Autodesk Inventor part; units mm, degrees
ref_plane "Plan de construction1" through (0, 5, 0) normal (0, -1, 0) x (1, 0, 0)
ref_plane "YZ Plane" through (0, 0, 0) normal (1, 0, 0) x (0, 1, 0)
ref_plane "XZ Plane" through (0, 0, 0) normal (0, 1, 0) x (-1, 0, 0)
sketch "Esquisse1" plane through (0, 0, 0) normal (0, 1, 0) x (-1, 0, 0)
  circle A0 centre (0, 0) radius 17.75
  dimension "d0" = 35.5
extrude "Extrusion1" add sketch "Esquisse1" along normal blind 8
ref_plane "Plan de construction1" through (0, 5, 0) normal (0, -1, 0) x (1, 0, 0)
sketch "Esquisse2" plane through (0, 5, 0) normal (0, -1, 0) x (1, 0, 0)
  circle A0 centre (0, 0) radius 17.75 construction
  line L0 (0, 0) -> (11, 0) construction
  circle A1 centre (11, 0) radius 1.65
  dimension "d4" = 11
  dimension "d5" = 3.3
extrude "Extrusion2" cut sketch "Esquisse2" along normal through all both and the other way through all
sketch "Esquisse3" plane through (0, 5, 0) normal (0, -1, 0) x (1, 0, 0)
  line L0 (23.2, 2.825) -> (8.2, 2.825)
  line L1 (8.2, 2.825) -> (8.2, -2.825)
  line L2 (8.2, -2.825) -> (23.2, -2.825)
  line L3 (23.2, -2.825) -> (23.2, 2.825)
  circle A0 centre (11, 0) radius 1.65 construction
  circle A1 centre (0, 0) radius 17.75 construction
  line L4 (0, 0) -> (8.2, 0) construction
  dimension "d8" = 5.65
  dimension "d9" = 2.8
  dimension "d10" = 15
pattern_circular "Réseau circulaire1" count 3 over 360 about axis through (0, 0, 0) along (0, -1, 0) of "Extrusion2"
ref_plane "Work Plane2" through (0, 6.5, 0) normal (0, 1, 0) x (1, 0, 0)
sketch "Sketch4" plane through (0, 6.5, 0) normal (0, 1, 0) x (1, 0, 0)
  circle A0 centre (0, 0) radius 17
  circle A1 centre (-5.5, -9.5263) radius 1.65
  circle A2 centre (11, 0) radius 1.65
  circle A3 centre (0, 0) radius 17.75
  circle A4 centre (0, 0) radius 17.75
  line L0 (-5.1051, -17) -> (-5.1051, 17)
  dimension "d17" = 34
extrude "Extrusion4" [suppressed]
sketch "Sketch7" plane through (0, 0, 0) normal (0, -1, 0) x (1, 0, 0)
  circle A0 centre (-5.5, -9.5263) radius 1.65
  circle A1 centre (-5.5, 9.5263) radius 1.65
  circle A2 centre (11, 0) radius 1.65
  circle A3 centre (0, 0) radius 17.75
  arc A4 (12.2653, -21.0869) -> (-1.702, -23.304) centre (6.3902, -29.1791) ccw construction
  line L0 (12.2653, -21.0869) -> (14.1974, -23.6673) construction
  arc A5 (16.0148, -22.871) -> (19.1393, -21.699) centre (17.1898, -21.2525) ccw construction
  arc A6 (19.1393, -21.699) -> (17.9505, 23.1047) centre (-68.5898, -1.6093) ccw construction
  arc A7 (17.9505, 23.1047) -> (14.8221, 24.7813) centre (15.9506, 23.1301) ccw construction
  line L1 (14.8221, 24.7813) -> (14.299, 23.7665) construction
  circle A8 centre (10.9719, 0.0309) radius 1.5
  circle A9 centre (12.314, 17.2549) radius 1.5
  circle A10 centre (12.3141, -17.2245) radius 1.5
  circle A11 centre (10.9719, -0.0082) radius 3
  circle A12 centre (10.9719, -0.0082) radius 1.5
  circle A13 centre (12.3141, -17.2245) radius 1.5
  circle A14 centre (12.3141, -17.2245) radius 1.5
  arc A15 (14.1974, -23.6673) -> (17.3392, -3.7967) centre (-72.5704, 0.2356) ccw
  arc A16 (17.3635, 3.6841) -> (14.299, 23.7665) centre (-72.5704, 0.2356) ccw
  circle A17 centre (0, 0) radius 17.75
  arc A18 (14.1974, -23.6673) -> (-0.0039, -17.75) centre (-0.0039, -37.75) ccw
  arc A19 (0, 17.75) -> (14.299, 23.7665) centre (0, 37.75) ccw
  circle A20 centre (-5.5, -9.5263) radius 1.65
  circle A21 centre (-5.5, 9.5263) radius 1.65
  circle A22 centre (11, 0) radius 1.65
  circle A23 centre (0, 0) radius 17.75
  dimension "d50" = 1.3141
  dimension "d51" = 17.2245
  dimension "d53" = 20
  dimension "d54" = 20
  dimension "d61" = 1.314
  dimension "d62" = 17.224
  dimension "d63" = 90
  dimension "d64" = 90
  dimension "d66" = 20
  dimension "d67" = 20
extrude "Extrusion5" add sketch "Sketch7" against normal blind 8 contours A3 A19 A16 | A15 A18 A3
sketch "Sketch8" plane through (0, 8, 0) normal (0, 1, 0) x (1, 0, 0)
  circle A0 centre (12.3141, 17.2245) radius 1.5
  circle A1 centre (12.314, -17.2549) radius 1.5
  circle A2 centre (-5.5, 9.5263) radius 1.65
  circle A3 centre (-5.5, -9.5263) radius 1.65
  circle A4 centre (11, 0) radius 1.65
  arc A5 (-0.0039, 17.75) -> (0, -17.75) centre (0, 0) ccw
  arc A6 (14.299, -23.7665) -> (0, -17.75) centre (0, -37.75) ccw
  arc A7 (14.299, -23.7665) -> (17.3635, -3.6841) centre (-72.5704, -0.2356) ccw
  arc A8 (17.3635, -3.6841) -> (17.3392, 3.7967) centre (0, 0) ccw
  arc A9 (17.3392, 3.7967) -> (14.1974, 23.6673) centre (-72.5704, -0.2356) ccw
  arc A10 (-0.0039, 17.75) -> (14.1974, 23.6673) centre (-0.0039, 37.75) ccw
  arc A11 (14.299, -23.7665) -> (0, -17.75) centre (0, -37.75) ccw
  arc A12 (14.8721, -21.5382) -> (13.3292, -20.2477) centre (0, -37.75) ccw
  arc A13 (12.6827, -1.3087) -> (12.7364, 0.5886) centre (0, 0) ccw
  arc A14 (10.3425, 14.4255) -> (10.6571, 14.5677) centre (-0.0039, 37.75) ccw
  arc A15 (15.5707, -3.4578) -> (15.5479, 3.5588) centre (0, 0) ccw
  arc A16 (15.5479, 3.5588) -> (13.2545, 20.0947) centre (-72.5704, -0.2356) ccw
  arc A17 (17.3392, 3.7967) -> (14.1974, 23.6673) centre (-72.5704, -0.2356) ccw
  arc A18 (13.3292, -20.2477) -> (15.5707, -3.4578) centre (-72.5704, -0.2356) ccw
  arc A19 (11.9075, 19.0825) -> (11.9222, 19.0926) centre (-0.6265, 37.1628) ccw
  arc A20 (13.2545, 20.0947) -> (14.7767, 21.4548) centre (-0.6265, 37.1628) ccw
  dimension "d59" = 2
  dimension "d68" = 1.8
  dimension "d69" = 1.8
ref_plane "Work Plane3" through (0, 6.5, 0) normal (0, 1, 0) x (1, 0, 0)
ref_plane "Work Plane4" through (0, 1.5, 0) normal (0, -1, 0) x (1, 0, 0)
equation "\"d6\" = d5"
properties part number "capacitor_glue"
CAD build for the part. Positions are in the model's coordinates, mm. Round coordinates to 2 decimals unless told otherwise and drop trailing zeros. Write each loop counter-clockwise with the first axis right and the second up, starting at its lowest first coordinate (ties: lowest second). Pieces come first, ordered by that corner, then holes. Notation, with made-up numbers: (23.25, 50) -> (37.25, 50) arc R24 cw to (37.25, 71) -> close; hole circle Ø4 at (18, -21.5). An arc over 180 degrees is marked (long way). Answer in a Markdown table with one row per item. Add a question column.
Item 1: Saw through at B-B, the plane x = -5.5. Write the cut outline in (y, z).
Item 2: Mould opens along Z. For faces 1 (the face through (13.006, 3.944, -18.555)), 2 (the face through (7.65, 3.94, 19.27)), 3 (the face through (7.79, 3.94, -19.33)) say: pulls with the +Z half, pulls with the -Z half, needs draft (parallel to the pull), parting line crosses it, or undercut.
Item 3: Drop flat-ended pins along their axis: pin 1 Ø3 at (x, y) = (11, 1) entering from +Z; pin 2 Ø3 at (x, y) = (2.5, 2) entering from +Z; pin 3 Ø3 at (x, z) = (-5.5, 9.53) entering from +Y; pin 4 Ø1.5 at (x, y) = (1.5, 2) entering from -Z. Give the stop position or say it passes through.
Item 4: Saw through at D-D, the plane x = -10. Write the cut outline in (y, z) (3 decimals), then the cut area to 3 significant figures.
Item 5: Saw through at A-A, the plane z = 0. Write the cut outline in (x, y), then the cut area to 3 significant figures.
Item 6: Drill centre lines: line 1 (X direction, y = 4.5, z = 0); line 2 (Z direction, x = -5.5, y = 3.75); line 3 (Z direction, x = -0.5, y = 5.75). Where is each one in solid material? Low to high. Write a range as from..to.
Item 7: Saw through at C-C, the plane y = 6.5. Count the separate pieces of the cut face and the enclosed holes in it, then the cut area to 3 significant figures.
Findings below:
| question | item | result |
|---|---|---|
| 1 | outline | (0, -16.88) -> (8, -16.88) -> (8, -11.18) -> (0, -11.18) -> close; (0, -7.88) -> (8, -7.88) -> (8, 7.88) -> (0, 7.88) -> close; (0, 11.18) -> (8, 11.18) -> (8, 16.88) -> (0, 16.88) -> close |
| 2 | face 1 | undercut |
| 2 | face 2 | pulls with the +Z half |
| 2 | face 3 | pulls with the -Z half |
| 3 | pin 1 | stops at z = 22.14 |
| 3 | pin 2 | stops at z = 18.15 |
| 3 | pin 3 | passes through |
| 3 | pin 4 | stops at z = -17.88 |
| 4 | outline | (0, -14.665) -> (8, -14.665) -> (8, 14.665) -> (0, 14.665) -> close |
| 4 | area | 235 mm^2 |
| 5 | outline | (-17.75, 0) -> (9.35, 0) -> (9.35, 8) -> (-17.75, 8) -> close; (12.65, 0) -> (17.75, 0) -> (17.75, 8) -> (12.65, 8) -> close |
| 5 | area | 258 mm^2 |
| 6 | line 1 | x = -17.75..9.35, 12.65..17.75 |
| 6 | line 2 | z = -16.88..-11.18, -7.88..7.88, 11.18..16.88 |
| 6 | line 3 | z = -17.74..17.74 |
| 7 | separate pieces | 1 |
| 7 | enclosed holes | 5 |
| 7 | area | 1,120 mm^2 |
